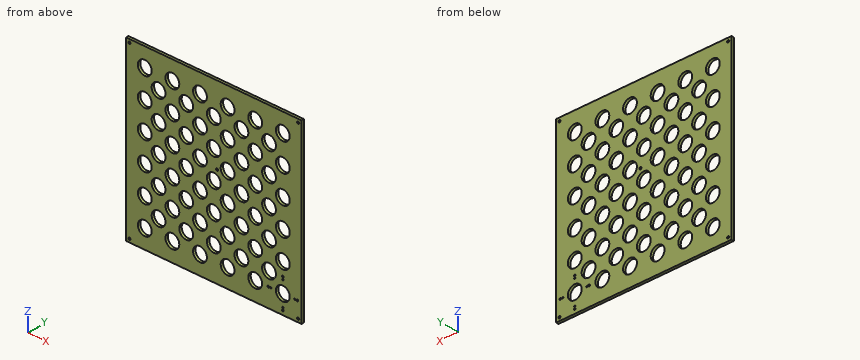
```python
from build123d import *

# Parameters (mm, degrees)
F0_W     = 800
F0_H     = 800
F0_R     = 31.5
F1_DEPTH = 12
F2_R     = 4
F2_R_2   = 3
F3_DEPTH = 12.001
F4_R     = 5
F5_DEPTH = 12.001


with BuildPart() as f1:
    # F0 (on Front) → F1 (new body)
    with BuildSketch(Plane.XZ):
        Rectangle(F0_W, F0_H)
        with Locations((-315, -315)):
            Circle(F0_R, mode=Mode.SUBTRACT)
        with Locations((-252, -252)):
            Circle(F0_R, mode=Mode.SUBTRACT)
        with Locations((-189, -315)):
            Circle(F0_R, mode=Mode.SUBTRACT)
        with Locations((-63, -315)):
            Circle(F0_R, mode=Mode.SUBTRACT)
        with Locations((-126, -252)):
            Circle(F0_R, mode=Mode.SUBTRACT)
        with Locations((-315, -189)):
            Circle(F0_R, mode=Mode.SUBTRACT)
        with Locations((-252, -126)):
            Circle(F0_R, mode=Mode.SUBTRACT)
        with Locations((-315, -63)):
            Circle(F0_R, mode=Mode.SUBTRACT)
        with Locations((-189, -189)):
            Circle(F0_R, mode=Mode.SUBTRACT)
        with Locations((-126, -126)):
            Circle(F0_R, mode=Mode.SUBTRACT)
        with Locations((-63, -189)):
            Circle(F0_R, mode=Mode.SUBTRACT)
        with Locations((-189, -63)):
            Circle(F0_R, mode=Mode.SUBTRACT)
        with Locations((-63, -63)):
            Circle(F0_R, mode=Mode.SUBTRACT)
        with Locations((63, -315)):
            Circle(F0_R, mode=Mode.SUBTRACT)
        with Locations((189, -315)):
            Circle(F0_R, mode=Mode.SUBTRACT)
        with Locations((0, -252)):
            Circle(F0_R, mode=Mode.SUBTRACT)
        with Locations((126, -252)):
            Circle(F0_R, mode=Mode.SUBTRACT)
        with Locations((315, -315)):
            Circle(F0_R, mode=Mode.SUBTRACT)
        with Locations((252, -252)):
            Circle(F0_R, mode=Mode.SUBTRACT)
        with Locations((63, -189)):
            Circle(F0_R, mode=Mode.SUBTRACT)
        with Locations((0, -126)):
            Circle(F0_R, mode=Mode.SUBTRACT)
        with Locations((189, -189)):
            Circle(F0_R, mode=Mode.SUBTRACT)
        with Locations((126, -126)):
            Circle(F0_R, mode=Mode.SUBTRACT)
        with Locations((63, -63)):
            Circle(F0_R, mode=Mode.SUBTRACT)
        with Locations((189, -63)):
            Circle(F0_R, mode=Mode.SUBTRACT)
        with Locations((252, -126)):
            Circle(F0_R, mode=Mode.SUBTRACT)
        with Locations((315, -189)):
            Circle(F0_R, mode=Mode.SUBTRACT)
        with Locations((315, -63)):
            Circle(F0_R, mode=Mode.SUBTRACT)
        with Locations((-315, 63)):
            Circle(F0_R, mode=Mode.SUBTRACT)
        with Locations((-252, 0)):
            Circle(F0_R, mode=Mode.SUBTRACT)
        with Locations((-315, 189)):
            Circle(F0_R, mode=Mode.SUBTRACT)
        with Locations((-252, 126)):
            Circle(F0_R, mode=Mode.SUBTRACT)
        with Locations((-126, 0)):
            Circle(F0_R, mode=Mode.SUBTRACT)
        with Locations((-189, 63)):
            Circle(F0_R, mode=Mode.SUBTRACT)
        with Locations((-63, 63)):
            Circle(F0_R, mode=Mode.SUBTRACT)
        with Locations((-126, 126)):
            Circle(F0_R, mode=Mode.SUBTRACT)
        with Locations((-189, 189)):
            Circle(F0_R, mode=Mode.SUBTRACT)
        with Locations((-63, 189)):
            Circle(F0_R, mode=Mode.SUBTRACT)
        with Locations((-252, 252)):
            Circle(F0_R, mode=Mode.SUBTRACT)
        with Locations((-315, 315)):
            Circle(F0_R, mode=Mode.SUBTRACT)
        with Locations((-126, 252)):
            Circle(F0_R, mode=Mode.SUBTRACT)
        with Locations((-189, 315)):
            Circle(F0_R, mode=Mode.SUBTRACT)
        with Locations((-63, 315)):
            Circle(F0_R, mode=Mode.SUBTRACT)
        Circle(F0_R, mode=Mode.SUBTRACT)
        with Locations((63, 63)):
            Circle(F0_R, mode=Mode.SUBTRACT)
        with Locations((126, 0)):
            Circle(F0_R, mode=Mode.SUBTRACT)
        with Locations((189, 63)):
            Circle(F0_R, mode=Mode.SUBTRACT)
        with Locations((0, 126)):
            Circle(F0_R, mode=Mode.SUBTRACT)
        with Locations((63, 189)):
            Circle(F0_R, mode=Mode.SUBTRACT)
        with Locations((126, 126)):
            Circle(F0_R, mode=Mode.SUBTRACT)
        with Locations((189, 189)):
            Circle(F0_R, mode=Mode.SUBTRACT)
        with Locations((252, 0)):
            Circle(F0_R, mode=Mode.SUBTRACT)
        with Locations((315, 63)):
            Circle(F0_R, mode=Mode.SUBTRACT)
        with Locations((252, 126)):
            Circle(F0_R, mode=Mode.SUBTRACT)
        with Locations((315, 189)):
            Circle(F0_R, mode=Mode.SUBTRACT)
        with Locations((0, 252)):
            Circle(F0_R, mode=Mode.SUBTRACT)
        with Locations((126, 252)):
            Circle(F0_R, mode=Mode.SUBTRACT)
        with Locations((63, 315)):
            Circle(F0_R, mode=Mode.SUBTRACT)
        with Locations((189, 315)):
            Circle(F0_R, mode=Mode.SUBTRACT)
        with Locations((252, 252)):
            Circle(F0_R, mode=Mode.SUBTRACT)
        with Locations((315, 315)):
            Circle(F0_R, mode=Mode.SUBTRACT)
    extrude(amount=F1_DEPTH)

    # F2 (on Front) → F3 (cut, through all)
    with BuildSketch(Plane.XZ):
        with Locations((315, -381)):
            Circle(F2_R)
        with Locations((381, -315)):
            Circle(F2_R)
        with Locations((315, -249)):
            Circle(F2_R)
        with Locations((249, -315)):
            Circle(F2_R)
        with Locations((315, -370)):
            Circle(F2_R_2)
        with Locations((370, -315)):
            Circle(F2_R_2)
        with Locations((315, -260)):
            Circle(F2_R_2)
        with Locations((260, -315)):
            Circle(F2_R_2)
    extrude(amount=F3_DEPTH, mode=Mode.SUBTRACT)

    # F4 (on Front) → F5 (cut, through all)
    with BuildSketch(Plane.XZ):
        with Locations((-385, -385)):
            Circle(F4_R)
        with Locations((-385, 385)):
            Circle(F4_R)
        with Locations((385, -385)):
            Circle(F4_R)
        with Locations((385, 385)):
            Circle(F4_R)
        with Locations((15, 50)):
            Circle(F4_R)
    extrude(amount=F5_DEPTH, mode=Mode.SUBTRACT)


solid = f1.part
```
Part model, mm, in its own coordinate system. Round coordinates to 2 decimals unless told otherwise and drop trailing zeros. Loops run counter-clockwise (first coordinate to the right, second up) from the corner with the lowest first, then second, coordinate; pieces in that order, holes last.
1. Slice it at B-B (z = 126). Give the cut face in (x, y), and give its area (3 significant figures).
Solutions:
outline: (-400, -12) - (-283.5, -12) - (-283.5, 0) - (-400, 0) - close; (-220.5, -12) - (-157.5, -12) - (-157.5, 0) - (-220.5, 0) - close; (-94.5, -12) - (-31.5, -12) - (-31.5, 0) - (-94.5, 0) - close; (31.5, -12) - (94.5, -12) - (94.5, 0) - (31.5, 0) - close; (157.5, -12) - (220.5, -12) - (220.5, 0) - (157.5, 0) - close; (283.5, -12) - (400, -12) - (400, 0) - (283.5, 0) - close
area: 5,820 mm2
2. Drill centre lines: line 1 along Z through (x, y) = (126, -7.5); line 2 along X through (y, z) = (-2, -240.5); line 3 along Z through (x, y) = (23, -2). Where is each one in solid material? Low to high.
Solutions:
line 1: z = -400 to -283.5, -220.5 to -157.5, -94.5 to -31.5, 31.5 to 94.5, 157.5 to 220.5, 283.5 to 400
line 2: x = -400 to -281.33, -222.67 to -155.33, -96.67 to -29.33, 29.33 to 96.67, 155.33 to 222.67, 281.33 to 400
line 3: z = -400 to -273.52, -230.48 to -147.52, -104.48 to -21.52, 21.52 to 104.48, 147.52 to 230.48, 273.52 to 400
3. Slice it at A-A (z = -189). Give the cut face in (x, y).
Solutions:
outline: (-400, -12) - (-346.5, -12) - (-346.5, 0) - (-400, 0) - close; (-283.5, -12) - (-220.5, -12) - (-220.5, 0) - (-283.5, 0) - close; (-157.5, -12) - (-94.5, -12) - (-94.5, 0) - (-157.5, 0) - close; (-31.5, -12) - (31.5, -12) - (31.5, 0) - (-31.5, 0) - close; (94.5, -12) - (157.5, -12) - (157.5, 0) - (94.5, 0) - close; (220.5, -12) - (283.5, -12) - (283.5, 0) - (220.5, 0) - close; (346.5, -12) - (400, -12) - (400, 0) - (346.5, 0) - close
4. Slice it at C-C (x = -67.5). Give the cut face in (y, z).
Solutions:
outline: (-12, -400) - (0, -400) - (0, -346.18) - (-12, -346.18) - close; (-12, -283.82) - (0, -283.82) - (0, -220.18) - (-12, -220.18) - close; (-12, -157.82) - (0, -157.82) - (0, -94.18) - (-12, -94.18) - close; (-12, -31.82) - (0, -31.82) - (0, 31.82) - (-12, 31.82) - close; (-12, 94.18) - (0, 94.18) - (0, 157.82) - (-12, 157.82) - close; (-12, 220.18) - (0, 220.18) - (0, 283.82) - (-12, 283.82) - close; (-12, 346.18) - (0, 346.18) - (0, 400) - (-12, 400) - close
5. Slice it at D-D (x = -238). Give the cut face in (y, z).
Solutions:
outline: (-12, -400) - (0, -400) - (0, -280.22) - (-12, -280.22) - close; (-12, -223.78) - (0, -223.78) - (0, -154.22) - (-12, -154.22) - close; (-12, -97.78) - (0, -97.78) - (0, -28.22) - (-12, -28.22) - close; (-12, 28.22) - (0, 28.22) - (0, 97.78) - (-12, 97.78) - close; (-12, 154.22) - (0, 154.22) - (0, 223.78) - (-12, 223.78) - close; (-12, 280.22) - (0, 280.22) - (0, 400) - (-12, 400) - close
